```python
from build123d import *

# Parameters (mm, degrees)
BOSS_EXTRU_1_START      = -15
BOSS_EXTRU_1_DEPTH      = 15
ENL_V_START             = -20
ENL_V_MAT_EXTRU_1_DEPTH = 20


with BuildPart() as part:
    # Esquisse2 → Révolution1 (revolve)
    with BuildSketch(Plane.XY):
        Polygon((0, 0), (0, 3.9), (25, 3.9), (25, 9.1), (45, 9.1), (45, 3.1), (32, 3.1), (30, 0), align=None)
    revolve(axis=Axis((30, 0, 0), (-1, 0, 0)))

    # Esquisse3 → Révolution2 (revolve)
    with BuildSketch(Plane.XY, mode=Mode.PRIVATE) as r_volution2_sk:
        Polygon((25, 3.9), (20, 3.9), (25, 9.1), align=None)
    revolve(r_volution2_sk.sketch.rotate(Axis((0, 0, 0), (1, 0, 0)), 90), axis=Axis((0, 0, 0), (1, 0, 0)))

    # Esquisse4 → Boss.-Extru.1 (add)
    with BuildSketch(Plane(origin=(45, 0, 0), x_dir=(0, 0, -1), z_dir=(1, 0, 0)).offset(BOSS_EXTRU_1_START)):
        with BuildLine():
            ThreePointArc((1.899341991, 2.45), (0, 3.1), (-1.899341991, 2.45))
            Line((-1.899341991, 2.45), (1.899341991, 2.45))
        make_face()
    extrude(amount=BOSS_EXTRU_1_DEPTH)

    # Esquisse5 → Enlèv. mat.-Extru.1 (cut)
    with BuildSketch(Plane.ZY.offset(ENL_V_START)):
        with BuildLine():
            ThreePointArc((2.491987159, 3), (0, 3.9), (-2.491987159, 3))
            Line((-2.491987159, 3), (2.491987159, 3))
        make_face()
    extrude(amount=ENL_V_MAT_EXTRU_1_DEPTH, mode=Mode.SUBTRACT)

    # Congé2: read off the stored shape, not the designer's step
    # Congé2 outline → Congé2 (revolve, cut)
    with BuildSketch(Plane.YX):
        with BuildLine():
            Line((3.9, 0), (3.9, 1))
            ThreePointArc((3.9, 1), (3.607106781, 0.292893219), (2.9, 0))
            Line((2.9, 0), (3.9, 0))
        make_face()
    revolve(axis=Axis((0, 0, 0), (1, 0, 0)), mode=Mode.SUBTRACT)


solid = part.part
```
Verification items for the finished model (mm, model axes). A direction names the side the tool comes from. Round coordinates to 2 decimals unless told otherwise and drop trailing zeros. Order: outer loops, then holes, each group sorted by start corner. A loop starts at its lowest first (then second) coordinate and runs counter-clockwise, first axis right, second up. Notation, with made-up numbers: (-20.75, 82) - (14.25, 82) arc R16 cw to (14.25, 93) - close; hole circle Ø3 at (-1, 78.25). An arc over 180 degrees is marked (long way). Use CSV: the item, a comma, the result in double quotes.
(1) Access from +Z, -Z, +X, -X, +Y, -Y to the whole of each face (thin tool, end or side, straight path). Record for faces 5 (the face through (35.14, -1.973, 8.884)), 6 (the face through (20, 3.4, 0)).
Entries:
face 5,"+X, -X"
face 6,"+Z, -Z, -X, +Y"
(2) Section check C-C on x = 12.5. Record the boundary of the cut face in (y, z).
Entries:
outline,"(3, -2.49) - (3, 2.49) arc R3.9 ccw (long way) to start"
(3) Section check B-B on x = 29. Record the boundary of the cut face in (y, z).
Entries:
outline,"circle Ø18.2 at (0, 0)"
(4) Section check A-A on x = 35. Record the boundary of the cut face in (y, z), and give its area (3 significant figures).
Entries:
outline,"circle Ø18.2 at (0, 0); hole (2.45, -1.9) - (2.45, 1.9) arc R3.1 ccw (long way) to start"
area,"232 mm^2"
(5) Mould release check, pull along Z, two halves, no side actions. Record for faces 1 (the face through (38, 2.45, 0)), 2 (the face through (10.6, -3.9, -0.1)), 3 (the face through (38.4, -3.1, -0.1)), 4 (the face through (45, -4, 0)): released by +Z, released by -Z, zero draft, split by the parting line, or undercut.
Entries:
face 1,"undercut"
face 2,"split by the parting line"
face 3,"undercut"
face 4,"zero draft"
(6) Gauge pin test, flat ends, axial feed: pin 1 Ø10 at (x, z) = (29, 7.5) entering from -Y; pin 2 Ø4 at (x, z) = (38, -3) entering from -Y; pin 3 Ø3.5 at (y, z) = (0, 0) entering from +X. Record the tip position at first contact, or that the pin passes through.
Entries:
pin 1,"y = -8.75"
pin 2,"y = -9.04"
pin 3,"x = 31.13"
(7) Thickness scan on probe 1 along Z at (x, y) = (36, 0); probe 2 along Y at (x, z) = (39.5, 0.25); probe 3 along Y at (x, z) = (36.5, 6.75). Record the ranges inside material, lowest first. Write a range as from..to.
Entries:
probe 1,"-9.1..-3.1, 3.1..9.1"
probe 2,"-9.1..-3.09, 2.45..9.1"
probe 3,"-6.1..6.1"
